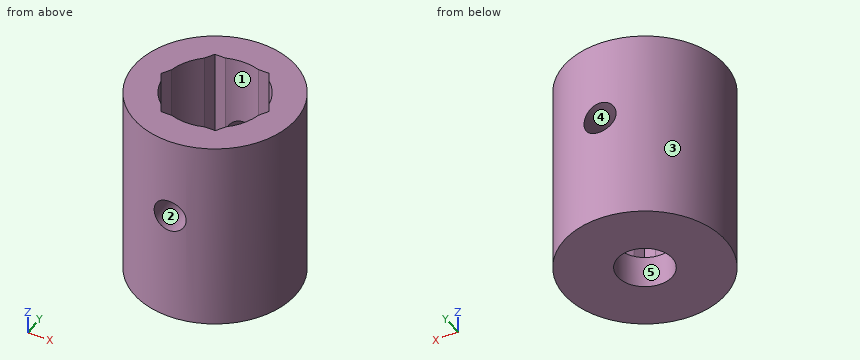
```python
from build123d import *

# Parameters (mm, degrees)
SKETCH1_R               = 5
BOSS_EXTRUDE1_DEPTH     = 6
SKETCH2_R               = 3
CUT_EXTRUDE1_DEPTH      = 10
CUT_EXTRUDE2_DEPTH      = 13.247448714
MOVE_START              = -4
MOVE_FACE1_DEPTH        = 10
MOVE_FACE2_DEPTH        = 10
SKETCH4_R               = 1.7
CUT_EXTRUDE3_DEPTH      = 14.928388277
CUT_EXTRUDE7_DEPTH      = 10.273618495
CUT_EXTRUDE7_DEPTH_BACK = 10.273618495
SKETCH10_R              = 1


# Read off the part's stored shape, not the designer's step: Move Face1, Move Face2
with BuildPart() as part:
    # Sketch1 → Boss-Extrude1 (new, symmetric)
    with BuildSketch(Plane.XY):
        Circle(SKETCH1_R)
    extrude(amount=BOSS_EXTRUDE1_DEPTH, both=True)

    # Sketch2 → Cut-Extrude1 (cut)
    with BuildSketch(Plane.XY.offset(6)):
        Circle(SKETCH2_R)
    extrude(amount=-CUT_EXTRUDE1_DEPTH, mode=Mode.SUBTRACT)

    # Sketch3 → Cut-Extrude2 (cut, through all)
    with BuildSketch(Plane.XY.offset(-4)):
        Polygon((1.573279484, 2.725), (-1.573279484, 2.725), (-3.146558967, 0), (-1.573279484, -2.725), (1.573279484, -2.725), (3.146558967, 0), align=None)
    extrude(amount=CUT_EXTRUDE2_DEPTH, mode=Mode.SUBTRACT)

    # Move Face1 outline → Move Face1 (cut)
    with BuildSketch(Plane.XY.offset(MOVE_START)):
        with BuildLine():
            Line((2.866431597, -0.885194838), (3.377499075, 0))
            Line((3.377499075, 0), (2.866431597, 0.885194838))
            ThreePointArc((2.866431597, 0.885194838), (2.942674777, 0.583665277), (2.98728973, 0.275862411))
            Line((2.98728973, 0.275862411), (3.146558967, 0))
            Line((3.146558967, 0), (2.98728973, -0.275862411))
            ThreePointArc((2.98728973, -0.275862411), (2.942674777, -0.583665277), (2.866431597, -0.885194838))
        make_face()
        with BuildLine():
            Line((1.688749537, -2.925), (2.199817015, -2.039805162))
            ThreePointArc((2.199817015, -2.039805162), (1.976806346, -2.256598473), (1.732548721, -2.449137589))
            Line((1.732548721, -2.449137589), (1.573279484, -2.725))
            Line((1.573279484, -2.725), (1.254741009, -2.725))
            ThreePointArc((1.254741009, -2.725), (0.965868431, -2.840263751), (0.666614581, -2.925))
            Line((0.666614581, -2.925), (1.688749537, -2.925))
        make_face()
        with BuildLine():
            ThreePointArc((1.732548721, 2.449137589), (1.976806346, 2.256598473), (2.199817015, 2.039805162))
            Line((2.199817015, 2.039805162), (1.688749537, 2.925))
            Line((1.688749537, 2.925), (0.666614581, 2.925))
            ThreePointArc((0.666614581, 2.925), (0.965868431, 2.840263751), (1.254741009, 2.725))
            Line((1.254741009, 2.725), (1.573279484, 2.725))
            Line((1.573279484, 2.725), (1.732548721, 2.449137589))
        make_face()
        with BuildLine():
            Line((-1.688749537, -2.925), (-0.666614581, -2.925))
            ThreePointArc((-0.666614581, -2.925), (-0.965868431, -2.840263751), (-1.254741009, -2.725))
            Line((-1.254741009, -2.725), (-1.573279484, -2.725))
            Line((-1.573279484, -2.725), (-1.732548721, -2.449137589))
            ThreePointArc((-1.732548721, -2.449137589), (-1.976806346, -2.256598473), (-2.199817015, -2.039805162))
            Line((-2.199817015, -2.039805162), (-1.688749537, -2.925))
        make_face()
        with BuildLine():
            ThreePointArc((-1.254741009, 2.725), (-0.965868431, 2.840263751), (-0.666614581, 2.925))
            Line((-0.666614581, 2.925), (-1.688749537, 2.925))
            Line((-1.688749537, 2.925), (-2.199817015, 2.039805162))
            ThreePointArc((-2.199817015, 2.039805162), (-1.976806346, 2.256598473), (-1.732548721, 2.449137589))
            Line((-1.732548721, 2.449137589), (-1.573279484, 2.725))
            Line((-1.573279484, 2.725), (-1.254741009, 2.725))
        make_face()
        with BuildLine():
            Line((-3.377499075, 0), (-2.866431597, -0.885194838))
            ThreePointArc((-2.866431597, -0.885194838), (-2.942674777, -0.583665277), (-2.98728973, -0.275862411))
            Line((-2.98728973, -0.275862411), (-3.146558967, 0))
            Line((-3.146558967, 0), (-2.98728973, 0.275862411))
            ThreePointArc((-2.98728973, 0.275862411), (-2.942674777, 0.583665277), (-2.866431597, 0.885194838))
            Line((-2.866431597, 0.885194838), (-3.377499075, 0))
        make_face()
    extrude(amount=MOVE_FACE1_DEPTH, mode=Mode.SUBTRACT)

    # Move Face2 outline → Move Face2 (cut)
    with BuildSketch(Plane.XY.offset(MOVE_START)):
        with BuildLine():
            Line((2.866431597, 0.885194838), (3.046538126, 0.573241179))
            ThreePointArc((3.046538126, 0.573241179), (2.684678752, 1.55), (2.019710487, 2.351758821))
            Line((2.019710487, 2.351758821), (2.199817015, 2.039805162))
            ThreePointArc((2.199817015, 2.039805162), (2.598076211, 1.5), (2.866431597, 0.885194838))
        make_face()
        with BuildLine():
            ThreePointArc((2.019710487, -2.351758821), (2.684678752, -1.55), (3.046538126, -0.573241179))
            Line((3.046538126, -0.573241179), (2.866431597, -0.885194838))
            ThreePointArc((2.866431597, -0.885194838), (2.598076211, -1.5), (2.199817015, -2.039805162))
            Line((2.199817015, -2.039805162), (2.019710487, -2.351758821))
        make_face()
        with BuildLine():
            Line((0.666614581, 2.925), (1.026827639, 2.925))
            ThreePointArc((1.026827639, 2.925), (0, 3.1), (-1.026827639, 2.925))
            Line((-1.026827639, 2.925), (-0.666614581, 2.925))
            ThreePointArc((-0.666614581, 2.925), (0, 3), (0.666614581, 2.925))
        make_face()
        with BuildLine():
            ThreePointArc((-1.026827639, -2.925), (0, -3.1), (1.026827639, -2.925))
            Line((1.026827639, -2.925), (0.666614581, -2.925))
            ThreePointArc((0.666614581, -2.925), (0, -3), (-0.666614581, -2.925))
            Line((-0.666614581, -2.925), (-1.026827639, -2.925))
        make_face()
        with BuildLine():
            Line((-2.199817015, 2.039805162), (-2.019710487, 2.351758821))
            ThreePointArc((-2.019710487, 2.351758821), (-2.684678752, 1.55), (-3.046538126, 0.573241179))
            Line((-3.046538126, 0.573241179), (-2.866431597, 0.885194838))
            ThreePointArc((-2.866431597, 0.885194838), (-2.598076211, 1.5), (-2.199817015, 2.039805162))
        make_face()
        with BuildLine():
            ThreePointArc((-3.046538126, -0.573241179), (-2.684678752, -1.55), (-2.019710487, -2.351758821))
            Line((-2.019710487, -2.351758821), (-2.199817015, -2.039805162))
            ThreePointArc((-2.199817015, -2.039805162), (-2.598076211, -1.5), (-2.866431597, -0.885194838))
            Line((-2.866431597, -0.885194838), (-3.046538126, -0.573241179))
        make_face()
    extrude(amount=MOVE_FACE2_DEPTH, mode=Mode.SUBTRACT)

    # Sketch4 → Cut-Extrude3 (cut, through all)
    with BuildSketch(Plane(origin=(0, 0, -6), x_dir=(-1, 0, 0), z_dir=(0, 0, -1))):
        Circle(SKETCH4_R)
    extrude(amount=-CUT_EXTRUDE3_DEPTH, mode=Mode.SUBTRACT)

    # Sketch10 → Cut-Extrude7 (cut, two sides: drawn at the far end of the back side and taken through both)
    with BuildSketch(Plane(origin=(0, 0, 0), x_dir=(1, 0, 0), z_dir=(0, 1, 0)).offset(-CUT_EXTRUDE7_DEPTH_BACK)):
        with Locations(Location((0, -0.9, 0), (0, 0, 270))):
            Circle(SKETCH10_R)
    extrude(amount=CUT_EXTRUDE7_DEPTH + CUT_EXTRUDE7_DEPTH_BACK, mode=Mode.SUBTRACT)


solid = part.part
```
Here's how the part is built. I have some questions about the finished solid (model axes, mm). Face numbers are marked on the shaded views. A direction names the side the tool comes from. Round coordinates to 2 decimals unless told otherwise and drop trailing zeros. Order: outer loops, then holes, each group sorted by start corner. A loop starts at its lowest first (then second) coordinate and runs counter-clockwise, first axis right, second up. Notation, with made-up numbers: (19.5, 39.5) -> (33.5, 39.5) arc R27 ccw to (33.5, 62.5) -> close; hole circle Ø8 at (22, 58). An arc over 180 degrees is marked (long way). Use a Markdown table: item, result. Add a question column.
(1) For the marked faces 1 and 2, which set-ups out of +Z, -Z, +X, -X, +Y, -Y let a thin tool reach every point of the face, with its end or its side?
(2) Suppose I cut it at B-B, the plane z = 2.25. Please give me the cut outline in (x, y) (1 decimal), and give its area (3 significant figures).
(3) For pin 1 Ø1.5 at (x, z) = (-4, -4) entering from -Y; pin 2 Ø4.5 at (x, y) = (0, 0) entering from -Z; pin 3 Ø0.5 at (x, z) = (-1.5, 1.5) entering from -Y; pin 4 Ø0.7 at (x, z) = (-1.5, 1.5) entering from +Y, each with a flat end and sliding along its axis, tell me the tip position at first contact or that it passes through.
(4) If we mould it in two halves opening along Y, with no side actions, what happens to the marked faces 3, 4 and 5? For each: released by +Y, released by -Y, zero draft, split by the parting line, or undercut.
(5) Suppose I cut it at C-C, the plane y = -1.25. Please give me the cut outline in (x, z), and give its area (3 significant figures).
(6) I need wall thicknesses on line 1 along Z through (x, y) = (0, 4.1); line 2 along Y through (x, z) = (0, -4.55); line 3 along Y through (x, z) = (-2.25, -3.75). Which ranges of each line are inside material? Lowest first, please.
(7) Suppose I cut it at D-D, the plane x = 1.5. Please give me the cut outline in (y, z) (3 decimals), and give its area (3 significant figures).
(8) Suppose I cut it at A-A, the plane x = 0. Please give me the cut outline in (y, z), and give its area (3 significant figures).
Verdict:
| question | item | result |
|---|---|---|
| 1 | face 1 | +Z |
| 1 | face 2 | +Y, -Y |
| 2 | outline | circle Ø10 at (0, 0); hole (-3.4, 0) -> (-3, -0.6) arc R3.1 ccw to (-2, -2.4) -> (-1.7, -2.9) -> (-1, -2.9) arc R3.1 ccw to (1, -2.9) -> (1.7, -2.9) -> (2, -2.4) arc R3.1 ccw to (3, -0.6) -> (3.4, 0) -> (3, 0.6) arc R3.1 ccw to (2, 2.4) -> (1.7, 2.9) -> (1, 2.9) arc R3.1 ccw to (-1, 2.9) -> (-1.7, 2.9) -> (-2, 2.4) arc R3.1 ccw to (-3, 0.6) -> close |
| 2 | area | 47.5 mm2 |
| 3 | pin 1 | y = -3.8 |
| 3 | pin 2 | z = -6 |
| 3 | pin 3 | y = -4.84 |
| 3 | pin 4 | y = 4.87 |
| 4 | face 3 | split by the parting line |
| 4 | face 4 | zero draft |
| 4 | face 5 | undercut |
| 5 | outline | (-4.84, -6) -> (-1.15, -6) -> (-1.15, -4) -> (-2.84, -4) -> (-2.84, 6) -> (-4.84, 6) -> close; (1.15, -6) -> (4.84, -6) -> (4.84, 6) -> (2.84, 6) -> (2.84, -4) -> (1.15, -4) -> close |
| 5 | area | 54.8 mm2 |
| 6 | line 1 | -6 to -0.1, 1.9 to 6 |
| 6 | line 2 | -5 to -1.7, 1.7 to 5 |
| 6 | line 3 | -4.47 to -2.13, 2.13 to 4.47 |
| 7 | outline | (-4.77, -6) -> (-0.8, -6) -> (-0.8, -4) -> (-2.925, -4) -> (-2.925, 6) -> (-4.77, 6) -> close; (0.8, -6) -> (4.77, -6) -> (4.77, 6) -> (2.925, 6) -> (2.925, -4) -> (0.8, -4) -> close |
| 7 | area | 52.8 mm2 |
| 8 | outline | (-5, -6) -> (-1.7, -6) -> (-1.7, -4) -> (-3.1, -4) -> (-3.1, -0.1) -> (-5, -0.1) -> close; (-5, 1.9) -> (-3.1, 1.9) -> (-3.1, 6) -> (-5, 6) -> close; (1.7, -6) -> (5, -6) -> (5, -0.1) -> (3.1, -0.1) -> (3.1, -4) -> (1.7, -4) -> close; (3.1, 1.9) -> (5, 1.9) -> (5, 6) -> (3.1, 6) -> close |
| 8 | area | 43.6 mm2 |
